Check sheet for the modelled part. Datum: model origin and axes. Units: mm. Face numbers are marked on the shaded views. A direction names the side the tool comes from. Give positions to 0.01 mm unless a question says otherwise; leave off trailing zeros. Loops run counter-clockwise (first coordinate to the right, second up) from the corner with the lowest first, then second, coordinate; pieces in that order, holes last. Notation, with made-up numbers: (-6.5, 40) - (24.5, 40) arc R18 ccw to (24.5, 64) - close; hole circle Ø6 at (27, -5.5). An arc over 180 degrees is marked (long way). Answer in a Markdown table with one row per item. Add a question column.
(1) Sectioned sample at B-B on x = 8.89. Enter the section's corners in (y, z), then the cut area to 3 significant figures.
(2) Sectioned sample at A-A on y = 30.48. Enter the section's corners in (x, z), then the cut area to 3 significant figures.
(3) Set-up check for the marked faces 5, 6 and 7: record each of +Z, -Z, +X, -X, +Y, -Y from which the full face is reachable in a straight line by a thin tool's end or side.
(4) Sectioned sample at C-C on z = -21. Enter the section's corners in (x, y) (3 decimals), then the cut area to 3 significant figures.
(5) Thickness scan on L1, parallel to X at y = 30.48, z = -19; L2, parallel to Y at x = 20.32, z = -6; L3, parallel to Z at x = 2.5, y = 34.5. Record the ranges inside material, lowest first.
(6) Sectioned sample at D-D on z = -9.5. Enter the section's corners in (x, y) (3 decimals), then the cut area to 3 significant figures.
(7) Go/stop test with flat-tipped pins: P1, Ø4.5, axis at x = 1.5, z = -10.5, coming from the +Y side (3 decimals); P2, Ø12, axis at y = 13.5, z = -6.5, coming from the +X side (3 decimals); P3, Ø6, axis at x = 17.5, z = -8, coming from the -Y side. Record where each tip stops, or that it passes through.
(8) Draft check along Z on the marked faces 1, 2, 3 and 4. Enter one of: released by +Z, released by -Z, zero draft, split by the parting line, or undercut.
from build123d import *

# Parameters (mm, degrees)
SKETCH1_W               = 23.876
SKETCH1_H               = 25.4
BOSS_EXTRUDE1_DEPTH     = 3.175
SKETCH2_W               = 25.4
SKETCH2_H               = 23.876
BOSS_EXTRUDE2_DEPTH     = 3.175
SKETCH3_W               = 25.4
SKETCH3_H               = 7.9629
SKETCH3_H_2             = 7.874
BOSS_EXTRUDE3_DEPTH     = 6.985
CUT_EXTRUDE1_DEPTH      = 50.796957497
CUT_EXTRUDE1_DEPTH_BACK = 50.796957497
SKETCH4_R               = 3.81
FILLET1_R               = 2.54
FILLET2_R               = 2.54
FILLET3_R               = 2.54


with BuildPart() as part:
    # Sketch1 → Boss-Extrude1 (new body)
    with BuildSketch(Plane(origin=(0, 0, 0), x_dir=(0, 0, -1), z_dir=(1, 0, 0))):
        with Locations((11.938, 12.7)):
            Rectangle(SKETCH1_W, SKETCH1_H)
    extrude(amount=BOSS_EXTRUDE1_DEPTH)

    # Sketch2 → Boss-Extrude2 (add)
    with BuildSketch(Plane(origin=(0, 25.4, 0), x_dir=(1, 0, 0), z_dir=(0, 1, 0))):
        with Locations((12.7, 11.938)):
            Rectangle(SKETCH2_W, SKETCH2_H)
    extrude(amount=BOSS_EXTRUDE2_DEPTH)

    # Sketch3 → Boss-Extrude3 (add)
    with BuildSketch(Plane(origin=(0, 28.575, 0), x_dir=(1, 0, 0), z_dir=(0, 1, 0))):
        with Locations((12.7, 3.98145)):
            Rectangle(SKETCH3_W, SKETCH3_H)
        with Locations((12.7, 19.939)):
            Rectangle(SKETCH3_W, SKETCH3_H_2)
    extrude(amount=BOSS_EXTRUDE3_DEPTH)

    # Sketch4 → Cut-Extrude1 (cut, two sides: drawn at the far end of the back side and taken through both)
    with BuildSketch(Plane.XY.offset(-CUT_EXTRUDE1_DEPTH_BACK)):
        with Locations((8.89, 30.48)):
            Circle(SKETCH4_R)
        with Locations((20.32, 30.48)):
            Circle(SKETCH4_R)
    extrude(amount=CUT_EXTRUDE1_DEPTH + CUT_EXTRUDE1_DEPTH_BACK, mode=Mode.SUBTRACT)

    # Fillet1
    fillet1_edges = [part.edges().sort_by_distance(p)[0] for p in [
        (0, 35.56, -3.98145),
        (0, 35.56, -19.939),
    ]]
    fillet(fillet1_edges, radius=FILLET1_R)

    # Fillet2
    fillet2_edges = [part.edges().sort_by_distance(p)[0] for p in [
        (25.4, 25.4, -11.938),
    ]]
    fillet(fillet2_edges, radius=FILLET2_R)

    # Fillet3
    fillet3_edges = [part.edges().sort_by_distance(p)[0] for p in [
        (25.4, 35.56, -3.98145),
        (25.4, 35.56, -19.939),
    ]]
    fillet(fillet3_edges, radius=FILLET3_R)


solid = part.part
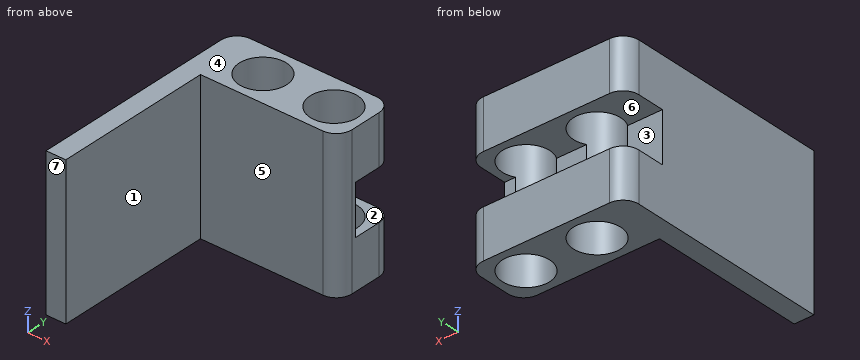
Reply:
| question | item | result |
|---|---|---|
| 1 | outline | (25.4, -23.88) - (26.67, -23.88) - (26.67, 0) - (25.4, 0) - close; (34.29, -23.88) - (35.56, -23.88) - (35.56, -16) - (34.29, -16) - close; (34.29, -7.96) - (35.56, -7.96) - (35.56, 0) - (34.29, 0) - close |
| 1 | area | 50.4 mm^2 |
| 2 | outline | (0, -23.88) - (5.08, -23.88) - (5.08, -16) - (0, -16) - close; (0, -7.96) - (5.08, -7.96) - (5.08, 0) - (0, 0) - close; (12.7, -23.88) - (16.51, -23.88) - (16.51, -16) - (12.7, -16) - close; (12.7, -7.96) - (16.51, -7.96) - (16.51, 0) - (12.7, 0) - close; (24.13, -23.88) - (25.4, -23.88) - (25.4, -16) - (24.13, -16) - close; (24.13, -7.96) - (25.4, -7.96) - (25.4, 0) - (24.13, 0) - close |
| 2 | area | 161 mm^2 |
| 3 | face 5 | +Z, -Z, +X, -Y |
| 3 | face 6 | +X, -X, +Y |
| 3 | face 7 | +Z, -Z, +X, -X, -Y |
| 4 | outline | (0, 0) - (3.175, 0) - (3.175, 25.4) - (22.86, 25.4) arc R2.54 ccw to (25.4, 27.94) - (25.4, 33.02) arc R2.54 ccw to (22.86, 35.56) - (2.54, 35.56) arc R2.54 ccw to (0, 33.02) - close; hole circle Ø7.62 at (8.89, 30.48); hole circle Ø7.62 at (20.32, 30.48) |
| 4 | area | 243 mm^2 |
| 5 | L1 | 0 to 5.08, 12.7 to 16.51, 24.13 to 25.4 |
| 5 | L2 | 25.4 to 26.67, 34.29 to 35.56 |
| 5 | L3 | -23.88 to -16, -7.96 to 0 |
| 6 | outline | (0, 0) - (3.175, 0) - (3.175, 25.4) - (22.86, 25.4) arc R2.54 ccw to (25.4, 27.94) - (25.4, 28.575) - (23.62, 28.575) arc R3.81 cw to (17.02, 28.575) - (12.19, 28.575) arc R3.81 cw to (5.59, 28.575) - (0, 28.575) - close |
| 6 | area | 142 mm^2 |
| 7 | P1 | y = 28.575 |
| 7 | P2 | x = 3.175 |
| 7 | P3 | y = 25.4 |
| 8 | face 1 | zero draft |
| 8 | face 2 | undercut |
| 8 | face 3 | undercut |
| 8 | face 4 | released by +Z |
